Here's how the part is built. I have some questions about the finished solid (model axes, mm). Face numbers are marked on the shaded views. A direction names the side the tool comes from. Coordinates: 2 decimals unless noted, no trailing zeros. Order: outer loops, then holes, each group sorted by start corner. A loop starts at its lowest first (then second) coordinate and runs counter-clockwise, first axis right, second up. Notation, with made-up numbers: (-39, -19.75) - (-12, -19.75) arc R18 cw to (-12, 8.25) - close; hole circle Ø10 at (81, 46.25). An arc over 180 degrees is marked (long way). Answer as CSV lines item,"result". Start each with the question number.
Q1. Thinking about a two-plate mould opening in Z: for the marked faces 5, 6 and 7, which applies, released by +Z, released by -Z, zero draft, split by the parting line, or undercut?
Q2. Suppose I cut it at B-B (x = 42.5). Please give me the cut outline in (y, z), then the cut area to 3 significant figures.
Q3. For the marked faces 1, 2, 3 and 4, which set-ups out of +Z, -Z, +X, -X, +Y, -Y let a thin tool reach every point of the face, with its end or its side?
Q4. I need wall thicknesses on line 1 (Y direction, x = 37, z = -7); line 2 (Z direction, x = -7, y = 21); line 3 (X direction, y = 14, z = -6.5). Which ranges of each line are inside material? Lowest first, please.
Q5. Suppose I cut it at C-C (y = 25.5). Please give me the cut outline in (x, z).
Q6. Suppose I cut it at D-D (z = 6). Please give me the cut outline in (x, y), then the cut area to 3 significant figures.
Q7. Suppose I cut it at A-A (z = -13). Please give me the cut outline in (x, y), then the cut area to 3 significant figures.
Q8. For pin 1 Ø7 at (y, z) = (18.5, -5.5) entering from +X; pin 2 Ø13 at (x, y) = (42.5, 17.5) entering from -Z; pin 3 Ø7.5 at (x, z) = (41.5, 3) entering from -Y, each with a flat end and sliding along its axis, tell me the tip position at first contact or that it passes through.
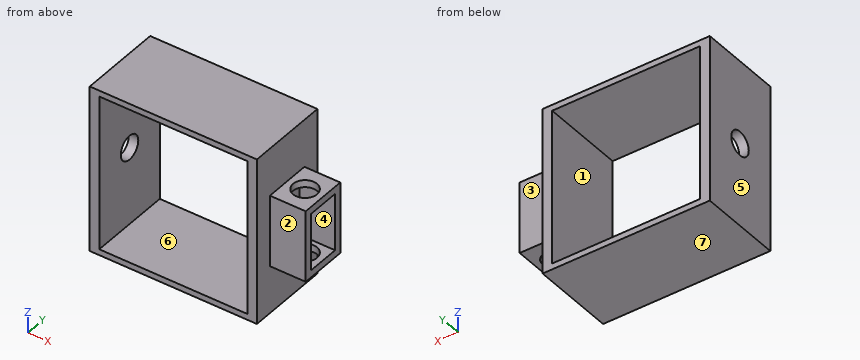
from build123d import *

# Parameters (mm, degrees)
SKETCH1_W           = 70
SKETCH1_H           = 70
BOSS_EXTRUDE1_DEPTH = 35
SKETCH2_W           = 62
SKETCH2_H           = 65
CUT_EXTRUDE1_DEPTH  = 61.621778265
SKETCH3_R           = 5.056768915
CUT_EXTRUDE2_DEPTH  = 15
SKETCH4_W           = 30
SKETCH4_H           = 20
BOSS_EXTRUDE2_DEPTH = 15
SKETCH6_W           = 24
SKETCH6_H           = 14
CUT_EXTRUDE3_DEPTH  = 15
SKETCH7_R           = 5.033880115
CUT_EXTRUDE4_DEPTH  = 79.89866919


with BuildPart() as part:
    # Sketch1 → Boss-Extrude1 (new body)
    with BuildSketch(Plane(origin=(0, 0, 0), x_dir=(1, 0, 0), z_dir=(0, 1, 0))):
        Rectangle(SKETCH1_W, SKETCH1_H)
    extrude(amount=BOSS_EXTRUDE1_DEPTH)

    # Sketch2 → Cut-Extrude1 (cut, through all)
    with BuildSketch(Plane(origin=(0, 35, 0), x_dir=(1, 0, 0), z_dir=(0, 1, 0))):
        Rectangle(SKETCH2_W, SKETCH2_H)
    extrude(amount=-CUT_EXTRUDE1_DEPTH, mode=Mode.SUBTRACT)

    # Sketch3 → Cut-Extrude2 (cut)
    with BuildSketch(Plane.ZY.offset(35)):
        with Locations((0, 17.5)):
            Circle(SKETCH3_R)
    extrude(amount=-CUT_EXTRUDE2_DEPTH, mode=Mode.SUBTRACT)

    # Sketch4 → Boss-Extrude2 (add)
    with BuildSketch(Plane(origin=(35, 0, 0), x_dir=(0, 0, -1), z_dir=(1, 0, 0))):
        with Locations((0, 17.5)):
            Rectangle(SKETCH4_W, SKETCH4_H)
    extrude(amount=BOSS_EXTRUDE2_DEPTH)

    # Sketch6 → Cut-Extrude3 (cut)
    with BuildSketch(Plane(origin=(50, 0, 0), x_dir=(0, 0, -1), z_dir=(1, 0, 0))):
        with Locations((0, 17.5)):
            Rectangle(SKETCH6_W, SKETCH6_H)
    extrude(amount=-CUT_EXTRUDE3_DEPTH, mode=Mode.SUBTRACT)

    # Sketch7 → Cut-Extrude4 (cut, through all)
    with BuildSketch(Plane.XY.offset(15)):
        with Locations((42.5, 17.5)):
            Circle(SKETCH7_R)
    extrude(amount=-CUT_EXTRUDE4_DEPTH, mode=Mode.SUBTRACT)


solid = part.part
Here are the results:
1,face 5,"zero draft"
1,face 6,"undercut"
1,face 7,"released by -Z"
2,outline,"(7.5, -15) - (12.47, -15) - (12.47, -12) - (10.5, -12) - (10.5, 12) - (12.47, 12) - (12.47, 15) - (7.5, 15) - close; (22.53, -15) - (27.5, -15) - (27.5, 15) - (22.53, 15) - (22.53, 12) - (24.5, 12) - (24.5, -12) - (22.53, -12) - close"
2,area,"204 mm²"
3,face 1,"+Y, -Y"
3,face 2,"+Z, -Z, +X, -Y"
3,face 3,"+Z, -Z, +X, +Y"
3,face 4,"+X"
4,line 1,"y = 7.5 to 10.5, 24.5 to 27.5"
4,line 2,"z = -35 to -32.5, 32.5 to 35"
4,line 3,"x = -35 to -31, 31 to 35"
5,outline,"(-35, -35) - (35, -35) - (35, -15) - (50, -15) - (50, 15) - (35, 15) - (35, 35) - (-35, 35) - close; hole (-31, -32.5) - (31, -32.5) - (31, 32.5) - (-31, 32.5) - close"
6,outline,"(-35, 0) - (-31, 0) - (-31, 35) - (-35, 35) - close; (31, 0) - (35, 0) - (35, 7.5) - (50, 7.5) - (50, 10.5) - (35, 10.5) - (35, 24.5) - (50, 24.5) - (50, 27.5) - (35, 27.5) - (35, 35) - (31, 35) - close"
6,area,"370 mm²"
7,outline,"(-35, 0) - (-31, 0) - (-31, 35) - (-35, 35) - close; (31, 0) - (35, 0) - (35, 7.5) - (50, 7.5) - (50, 27.5) - (35, 27.5) - (35, 35) - (31, 35) - close; hole circle Ø10.07 at (42.5, 17.5)"
7,area,"500 mm²"
8,pin 1,"stops at x = 35"
8,pin 2,"stops at z = -15"
8,pin 3,"stops at y = 7.5"
